Here's how the part is built. I have some questions about the finished solid (model axes, mm). A direction names the side the tool comes from. Give positions to 0.01 mm unless a question says otherwise; leave off trailing zeros. Loops run counter-clockwise (first coordinate to the right, second up) from the corner with the lowest first, then second, coordinate; pieces in that order, holes last. Notation, with made-up numbers: (5, 39) - (16, 39) arc R27 cw to (16, 76) - close; hole circle Ø4 at (9.5, 20.25). An arc over 180 degrees is marked (long way). Use one line per item in the form item = value.
from build123d import *

# Parameters (mm, degrees)
BOSS_EXTRUDE1_DEPTH = 914.4
SKETCH2_W           = 723.9
SKETCH2_H           = 50.8
CUT_EXTRUDE1_DEPTH  = 76.2
SKETCH2_2_W         = 723.9
SKETCH2_2_H         = 50.8
CUT_EXTRUDE2_DEPTH  = 25.4
SKETCH3_W           = 723.9
SKETCH3_H           = 41.992084525
CUT_EXTRUDE3_DEPTH  = 25.4


with BuildPart() as part:
    # Sketch1 → Boss-Extrude1 (new body)
    with BuildSketch(Plane(origin=(0, 0, 0), x_dir=(0, 0, -1), z_dir=(1, 0, 0))):
        Polygon((0, 0), (44.649353735, 0), (44.649353735, 171.45), (-18.850646265, 171.45), (-18.850646265, 69.85), (-8.690646265, 69.85), (7.184204897, 26.234204897), (0, 19.05), align=None)
    extrude(amount=BOSS_EXTRUDE1_DEPTH)

    # Sketch2 → Cut-Extrude1 (cut, along a direction that is not the sketch's normal)
    with BuildSketch(Plane.XY.offset(18.850646265)):
        with Locations((457.2, 139.7)):
            Rectangle(SKETCH2_W, SKETCH2_H)
    extrude(amount=-CUT_EXTRUDE1_DEPTH, dir=(0, 0.9396926207859081, 0.34202014332566966), mode=Mode.SUBTRACT)

    # Sketch2<2> → Cut-Extrude2 (cut)
    with BuildSketch(Plane.XY.offset(18.850646265)):
        with Locations((457.2, 139.7)):
            Rectangle(SKETCH2_2_W, SKETCH2_2_H)
    extrude(amount=-CUT_EXTRUDE2_DEPTH, mode=Mode.SUBTRACT)

    # Sketch3 → Cut-Extrude3 (cut)
    with BuildSketch(Plane(origin=(0, 5.377777955, -14.775323497), x_dir=(1, 0, 0), z_dir=(0, -0.34202014332566977, 0.9396926207859081))):
        with Locations((457.2, 47.613863381)):
            Rectangle(SKETCH3_W, SKETCH3_H)
    extrude(amount=-CUT_EXTRUDE3_DEPTH, mode=Mode.SUBTRACT)


solid = part.part
(1) If we section it at A-A (x = 493): List the corners of the cut face in (y, z) for me.
Geometry says:
outline = (0, -44.65) - (171.45, -44.65) - (171.45, 18.85) - (165.1, 18.85) - (165.1, -6.55) - (114.3, -6.55) - (114.3, 0.36) - (93.5, -7.21) - (75.64, -7.21) - (78.54, -15.18) - (39.08, -29.54) - (30.39, -5.67) - (26.23, -7.18) - (19.05, 0) - (0, 0) - close; (69.85, 8.69) - (71.78, 3.38) - (114.3, 18.85) - (69.85, 18.85) - close
(2) If we section it at B-B (y = 130.5): List the corners of the cut face in (x, z) for me.
Geometry says:
outline = (0, -44.65) - (914.4, -44.65) - (914.4, 18.85) - (819.15, 18.85) - (819.15, -6.55) - (95.25, -6.55) - (95.25, 18.85) - (0, 18.85) - close
(3) For faces 4 (the flat face through (452.133, 104.043, -3.372)), 5 (the flat face through (451, 110, 18.851)), 6 (the flat face through (455.066, 27.144, -6.853)), 7 (the flat face through (452, 140, -6.549)), which set-ups out of +Z, -Z, +X, -X, +Y, -Y let a thin tool reach every point of the face, with its end or its side?
Geometry says:
face_4 = none
face_5 = +Z, +X, -X, +Y, -Y
face_6 = +Z, +X, -X
face_7 = +Z
(4) For P1, Ø5, axis at x = 137.5, y = 45.5, coming from the +Z side; P2, Ø8, axis at x = 477, y = 137.5, coming from the +Z side; P3, Ø15, axis at x = 337.5, y = 6.5, coming from the +Z side, each with a flat end and sliding along its axis, tell me the tip position at first contact or that it passes through.
Geometry says:
P1 = -26.29
P2 = -6.55
P3 = 0
(5) If we section it at C-C (x = 839): List the corners of the cut face in (y, z) for me.
Geometry says:
outline = (0, -44.65) - (171.45, -44.65) - (171.45, 18.85) - (69.85, 18.85) - (69.85, 8.69) - (26.23, -7.18) - (19.05, 0) - (0, 0) - close
(6) If I drill on probe 1 along X at (y, z) = (146, -5.5); probe 2 along Z at (x, y) = (664.5, 153); probe 3 along Y at (x, z) = (162.5, -11), over which ranges is the centre line in solid material (lowest first)?
Geometry says:
probe_1 = 0 to 95.25, 819.15 to 914.4
probe_2 = -44.65 to -6.55
probe_3 = 0 to 32.33, 77.02 to 171.45
(7) Thinking about a two-plate mould opening in Y: for faces 1 (the flat face through (452, 165.1, 6)), 2 (the flat face through (451, 0, -22)), 3 (the flat face through (451, 10, 0)), which applies, pulls with the +Y half, pulls with the -Y half, needs draft (parallel to the pull), parting line crosses it, or undercut?
Geometry says:
face_1 = undercut
face_2 = pulls with the -Y half
face_3 = needs draft
